Model file for the job. Use its own axes, mm. A direction names the side the tool comes from. Round coordinates to 2 decimals unless told otherwise and drop trailing zeros. Write each loop counter-clockwise with the first axis right and the second up, starting at its lowest first coordinate (ties: lowest second). Pieces come first, ordered by that corner, then holes. Notation, with made-up numbers: (47, 57) - (54, 57) arc R17 ccw to (54, 87) - close; hole circle Ø9 at (58.25, 47.5). An arc over 180 degrees is marked (long way). One line per item, written item: value.
from build123d import *

# Parameters (mm, degrees)
CROQUIS1_W                   = 36
CROQUIS1_H                   = 34
SALIENTE_EXTRUIR1_DEPTH      = 1.5
CROQUIS2_W                   = 15
CROQUIS2_H                   = 5
CORTAR_EXTRUIR1_DEPTH        = 1.5
CROQUIS3_R                   = 1.5875
CORTAR_EXTRUIR2_DEPTH        = 2.54
CROQUIS4_W                   = 34
CROQUIS4_H                   = 23
SALIENTE_EXTRUIR2_DEPTH      = 2
CROQUIS5_W                   = 32
CROQUIS5_H                   = 17
SALIENTE_EXTRUIR5_DEPTH      = 0.1
SALIENTE_EXTRUIR7_DEPTH      = 2
SALIENTE_EXTRUIR7_DEPTH_BACK = 10
CROQUIS15_W                  = 1
CROQUIS15_H                  = 1
CROQUIS16_W                  = 2
CROQUIS16_H                  = 2
SALIENTE_EXTRUIR8_DEPTH      = 2
CROQUIS17_W                  = 9.62
CROQUIS17_H                  = 1.5
SALIENTE_EXTRUIR9_DEPTH      = 2
REDONDEO1_R                  = 0.5
CROQUIS41_R                  = 2.0875
CORTAR_EXTRUIR4_DEPTH        = 0.01
CORTAR_EXTRUIR5_START        = -0.01
CROQUIS42_R                  = 2.0875
CORTAR_EXTRUIR5_DEPTH        = 0.01


with BuildPart() as part:
    # Croquis1 → Saliente-Extruir1 (new body)
    with BuildSketch(Plane.XY):
        Rectangle(CROQUIS1_W, CROQUIS1_H)
    extrude(amount=SALIENTE_EXTRUIR1_DEPTH)

    # Croquis2 → Cortar-Extruir1 (cut)
    with BuildSketch(Plane.XY.offset(1.5)):
        with Locations((0, 14.5)):
            Rectangle(CROQUIS2_W, CROQUIS2_H)
    extrude(amount=-CORTAR_EXTRUIR1_DEPTH, mode=Mode.SUBTRACT)

    # Croquis3 → Cortar-Extruir2 (cut)
    with BuildSketch(Plane.XY.offset(1.5)):
        with Locations((-15.4125, 14.2875)):
            Circle(CROQUIS3_R)
        with Locations((15.4125, 14.2875)):
            Circle(CROQUIS3_R)
        with Locations((15.4125, -14.2875)):
            Circle(CROQUIS3_R)
        with Locations((-15.4125, -14.2875)):
            Circle(CROQUIS3_R)
    extrude(amount=-CORTAR_EXTRUIR2_DEPTH, mode=Mode.SUBTRACT)

    # Croquis4 → Saliente-Extruir2 (add)
    with BuildSketch(Plane.XY.offset(1.5)):
        with Locations((0, 0.3)):
            Rectangle(CROQUIS4_W, CROQUIS4_H)
    extrude(amount=SALIENTE_EXTRUIR2_DEPTH)

    # Croquis5 → Saliente-Extruir5 (add)
    with BuildSketch(Plane.XY.offset(3.5)):
        with Locations((0, -1.7)):
            Rectangle(CROQUIS5_W, CROQUIS5_H)
    extrude(amount=SALIENTE_EXTRUIR5_DEPTH)

    # Croquis15 → Saliente-Extruir7 (add, two sides: drawn at the far end of the back side and taken through both)
    with BuildSketch(Plane.XY.offset(1.5).offset(-SALIENTE_EXTRUIR7_DEPTH_BACK)):
        with Locations((1.27, -15.75)):
            Rectangle(CROQUIS15_W, CROQUIS15_H)
        with Locations((3.81, -15.75)):
            Rectangle(CROQUIS15_W, CROQUIS15_H)
        with Locations((-1.27, -15.75)):
            Rectangle(CROQUIS15_W, CROQUIS15_H)
        with Locations((-3.81, -15.75)):
            Rectangle(CROQUIS15_W, CROQUIS15_H)
    extrude(amount=SALIENTE_EXTRUIR7_DEPTH + SALIENTE_EXTRUIR7_DEPTH_BACK)

    # Croquis16 → Saliente-Extruir8 (add)
    with BuildSketch(Plane(origin=(0, 0, 0), x_dir=(-1, 0, 0), z_dir=(0, 0, -1))):
        with Locations((3.81, -15.75)):
            Rectangle(CROQUIS16_W, CROQUIS16_H)
        with Locations((1.27, -15.75)):
            Rectangle(CROQUIS16_W, CROQUIS16_H)
        with Locations((-1.27, -15.75)):
            Rectangle(CROQUIS16_W, CROQUIS16_H)
        with Locations((-3.81, -15.75)):
            Rectangle(CROQUIS16_W, CROQUIS16_H)
    extrude(amount=SALIENTE_EXTRUIR8_DEPTH)

    # Croquis17 → Saliente-Extruir9 (add)
    with BuildSketch(Plane(origin=(0, 0, 0), x_dir=(-1, 0, 0), z_dir=(0, 0, -1))):
        with Locations((0, -15.75)):
            Rectangle(CROQUIS17_W, CROQUIS17_H)
    extrude(amount=SALIENTE_EXTRUIR9_DEPTH)

    # Redondeo1
    redondeo1_edges = [part.edges().sort_by_distance(p)[0] for p in [
        (0.77, -15.75, 1.5),
        (1.27, -15.25, 1.5),
        (1.77, -15.75, 1.5),
        (1.27, -16.25, 1.5),
        (-1.77, -15.75, 1.5),
        (-1.27, -15.25, 1.5),
        (-0.77, -15.75, 1.5),
        (-1.27, -16.25, 1.5),
        (-4.31, -15.75, 1.5),
        (-3.81, -15.25, 1.5),
        (-3.31, -15.75, 1.5),
        (-3.81, -16.25, 1.5),
        (3.31, -15.75, 1.5),
        (3.81, -15.25, 1.5),
        (4.31, -15.75, 1.5),
        (3.81, -16.25, 1.5),
    ]]
    fillet(redondeo1_edges, radius=REDONDEO1_R)

    # Croquis41 → Cortar-Extruir4 (cut)
    with BuildSketch(Plane.XY.offset(1.5)):
        with Locations((-15.4125, 14.2875)):
            Circle(CROQUIS41_R)
        with Locations((15.4125, 14.2875)):
            Circle(CROQUIS41_R)
        with Locations((15.4125, -14.2875)):
            Circle(CROQUIS41_R)
        with Locations((-15.4125, -14.2875)):
            Circle(CROQUIS41_R)
    extrude(amount=-CORTAR_EXTRUIR4_DEPTH, mode=Mode.SUBTRACT)

    # Croquis42 → Cortar-Extruir5 (cut)
    with BuildSketch(Plane(origin=(0, 0, 0), x_dir=(-1, 0, 0), z_dir=(0, 0, -1)).offset(CORTAR_EXTRUIR5_START)):
        with Locations(Location((-15.4125, 14.2875, 0), (0, 0, 180))):
            Circle(CROQUIS42_R)
        with Locations(Location((15.4125, 14.2875, 0), (0, 0, 180))):
            Circle(CROQUIS42_R)
        with Locations(Location((15.4125, -14.2875, 0), (0, 0, 180))):
            Circle(CROQUIS42_R)
        with Locations(Location((-15.4125, -14.2875, 0), (0, 0, 180))):
            Circle(CROQUIS42_R)
    extrude(amount=CORTAR_EXTRUIR5_DEPTH, mode=Mode.SUBTRACT)


solid = part.part
1. Band-saw the part on B-B on y = -13.5. State how many separate pieces and enclosed holes the cut face has, plus the area to 3 significant figures.
Report:
separate pieces: 3
enclosed holes: 0
area: 45.7 mm²
2. Band-saw the part on D-D on x = 10. Write the cut outline in (y, z), plus the area to 3 significant figures.
Report:
outline: (-17, 0) - (17, 0) - (17, 1.5) - (11.8, 1.5) - (11.8, 3.5) - (6.8, 3.5) - (6.8, 3.6) - (-10.2, 3.6) - (-10.2, 3.5) - (-11.2, 3.5) - (-11.2, 1.5) - (-17, 1.5) - close
area: 98.7 mm²
3. Wall check: probe 1 along Z at (x, y) = (-14, 2); probe 2 along Y at (x, z) = (-9.5, 3); probe 3 along Z at (x, y) = (-2, -11.5). Give the ranges that are in metal, low to high. Write a range as [from, to].
Report:
probe 1: [0, 3.6]
probe 2: [-11.2, 11.8]
probe 3: [0, 1.5]
4. Band-saw the part on A-A on z = -3. Write the cut outline in (x, y).
Report:
outline: (-4.31, -16.25) - (-3.31, -16.25) - (-3.31, -15.25) - (-4.31, -15.25) - close; (-1.77, -16.25) - (-0.77, -16.25) - (-0.77, -15.25) - (-1.77, -15.25) - close; (0.77, -16.25) - (1.77, -16.25) - (1.77, -15.25) - (0.77, -15.25) - close; (3.31, -16.25) - (4.31, -16.25) - (4.31, -15.25) - (3.31, -15.25) - close
5. Drop flat-ended pins along their axis: pin 1 (0.8 mm diameter, centred on y = -15.5, z = 2.5, fed in from +X); pin 2 (1.9 mm diameter, centred on x = -15.41, y = 14.29, fed in from +Z); pin 3 (1.6 mm diameter, centred on x = -4, z = -1.5, fed in from +Y); pin 4 (6.5 mm diameter, centred on x = 15.41, y = -14.29, fed in from -Z). Give the stop position or say it passes through.
Report:
pin 1: x = 4.31
pin 2: through
pin 3: y = -14.75
pin 4: z = 0
6. Mould opens along Y. For faces 5 (the face through (0, -17, 1)), 6 (the face through (3.31, -16, -5)), 7 (the face through (-1, -15.25, 3)) say: released by +Y, released by -Y, zero draft, split by the parting line, or undercut.
Report:
face 5: released by -Y
face 6: zero draft
face 7: undercut
7. Band-saw the part on C-C on z = -0.5. Write the cut outline in (x, y).
Report:
outline: (-4.81, -16.75) - (-2.81, -16.75) - (-2.81, -16.5) - (-2.27, -16.5) - (-2.27, -16.75) - (-0.27, -16.75) - (-0.27, -16.5) - (0.27, -16.5) - (0.27, -16.75) - (2.27, -16.75) - (2.27, -16.5) - (2.81, -16.5) - (2.81, -16.75) - (4.81, -16.75) - (4.81, -14.75) - (2.81, -14.75) - (2.81, -15) - (2.27, -15) - (2.27, -14.75) - (0.27, -14.75) - (0.27, -15) - (-0.27, -15) - (-0.27, -14.75) - (-2.27, -14.75) - (-2.27, -15) - (-2.81, -15) - (-2.81, -14.75) - (-4.81, -14.75) - close
8. Tool access for faces 1 (the face through (3.31, -16, 3)), 2 (the face through (1, -16.75, -1)), 3 (the face through (4, -16, 3.5)), 4 (the face through (7.5, 14, 1)): list every direction of +Z, -Z, +X, -X, +Y, -Y with a clear straight run to the whole face (end or side of a thin tool).
Report:
face 1: +Z, -Y
face 2: -Z, +X, -X, -Y
face 3: +Z, +X, -X, -Y
face 4: +Z, -Z, +Y
